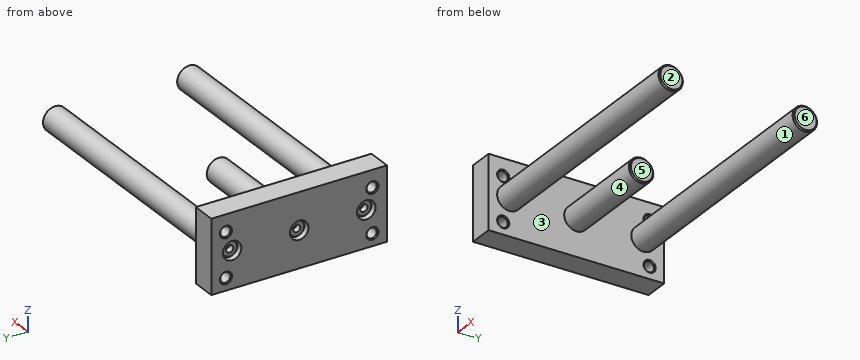
```python
from build123d import *

# Parameters (mm, degrees)
SKETCH1_W           = 30
SKETCH1_H           = 72
BOSS_EXTRUDE1_DEPTH = 10


with BuildPart() as part:
    # Sketch1 → Boss-Extrude1 (new body)
    with BuildSketch(Plane(origin=(0, 0, 0), x_dir=(0, 0, -1), z_dir=(1, 0, 0))):
        Rectangle(SKETCH1_W, SKETCH1_H)
    extrude(amount=BOSS_EXTRUDE1_DEPTH)

    # Sketch2 → Cut-Revolve1 (revolve, cut)
    with BuildSketch(Plane(origin=(0, 30, 0), x_dir=(-1, 0, 0), z_dir=(0, 1, 0)), mode=Mode.PRIVATE) as cut_revolve1_sk:
        Polygon((0, -10), (0, -12.5), (-0.433, -12.067), (-9.567, -12.067), (-10, -12.5), (-10, -10), align=None)
    revolve(cut_revolve1_sk.sketch.rotate(Axis((10, 30, -10), (-1, 0, 0)), 180), axis=Axis((10, 30, -10), (-1, 0, 0)), mode=Mode.SUBTRACT)

    # Sketch3 → Cut-Revolve2 (revolve, cut)
    with BuildSketch(Plane(origin=(0, 30, 0), x_dir=(-1, 0, 0), z_dir=(0, 1, 0)), mode=Mode.PRIVATE) as cut_revolve2_sk:
        Polygon((0, 8), (0, 5.5), (-0.433, 5.933), (-9.567, 5.933), (-10, 5.5), (-10, 8), align=None)
    revolve(cut_revolve2_sk.sketch.rotate(Axis((10, 30, 8), (-1, 0, 0)), 180), axis=Axis((10, 30, 8), (-1, 0, 0)), mode=Mode.SUBTRACT)

    # Sketch4 → Cut-Revolve3 (revolve, cut)
    with BuildSketch(Plane(origin=(0, -30, 0), x_dir=(-1, 0, 0), z_dir=(0, 1, 0)), mode=Mode.PRIVATE) as cut_revolve3_sk:
        Polygon((0, 8), (0, 5.5), (-0.433, 5.933), (-9.567, 5.933), (-10, 5.5), (-10, 8), align=None)
    revolve(cut_revolve3_sk.sketch.rotate(Axis((10, -30, 8), (-1, 0, 0)), 180), axis=Axis((10, -30, 8), (-1, 0, 0)), mode=Mode.SUBTRACT)

    # Sketch5 → Cut-Revolve4 (revolve, cut)
    with BuildSketch(Plane(origin=(0, -30, 0), x_dir=(-1, 0, 0), z_dir=(0, 1, 0)), mode=Mode.PRIVATE) as cut_revolve4_sk:
        Polygon((0, -10), (0, -12.5), (-0.433, -12.067), (-9.567, -12.067), (-10, -12.5), (-10, -10), align=None)
    revolve(cut_revolve4_sk.sketch.rotate(Axis((10, -30, -10), (-1, 0, 0)), 180), axis=Axis((10, -30, -10), (-1, 0, 0)), mode=Mode.SUBTRACT)

    # Sketch6 → Cut-Revolve5 (revolve, cut)
    with BuildSketch(Plane(origin=(0, 27.5, 0), x_dir=(-1, 0, 0), z_dir=(0, 1, 0)), mode=Mode.PRIVATE) as cut_revolve5_sk:
        Polygon((0, 0), (0, -3.8), (-5.555555556, -3.8), (-5.555555556, -3.5), (-2.055555556, -3.5), (-1.555555556, -3), (-1.555555556, -1.5), (-4.155555556, -1.5), (-5.021580959, 0), align=None)
    revolve(cut_revolve5_sk.sketch.rotate(Axis((5.021580959, 27.5, 0), (-1, 0, 0)), 180), axis=Axis((5.021580959, 27.5, 0), (-1, 0, 0)), mode=Mode.SUBTRACT)

    # Sketch7 → Cut-Revolve6 (revolve, cut)
    with BuildSketch(Plane(origin=(0, 0, 0), x_dir=(-1, 0, 0), z_dir=(0, 1, 0)), mode=Mode.PRIVATE) as cut_revolve6_sk:
        Polygon((0, 0), (0, -3.8), (-5.555555556, -3.8), (-5.555555556, -3.5), (-2.055555556, -3.5), (-1.555555556, -3), (-1.555555556, -1.5), (-4.155555556, -1.5), (-5.021580959, 0), align=None)
    revolve(cut_revolve6_sk.sketch.rotate(Axis((5.021580959, 0, 0), (-1, 0, 0)), 180), axis=Axis((5.021580959, 0, 0), (-1, 0, 0)), mode=Mode.SUBTRACT)

    # Sketch8 → Cut-Revolve7 (revolve, cut)
    with BuildSketch(Plane(origin=(0, -27.5, 0), x_dir=(-1, 0, 0), z_dir=(0, 1, 0)), mode=Mode.PRIVATE) as cut_revolve7_sk:
        Polygon((0, 0), (0, -3.8), (-5.555555556, -3.8), (-5.555555556, -3.5), (-2.055555556, -3.5), (-1.555555556, -3), (-1.555555556, -1.5), (-4.155555556, -1.5), (-5.021580959, 0), align=None)
    revolve(cut_revolve7_sk.sketch.rotate(Axis((5.021580959, -27.5, 0), (-1, 0, 0)), 180), axis=Axis((5.021580959, -27.5, 0), (-1, 0, 0)), mode=Mode.SUBTRACT)

    # Sketch9 → Revolve1 (revolve)
    with BuildSketch(Plane(origin=(0, 0, 0), x_dir=(-1, 0, 0), z_dir=(0, 1, 0)), mode=Mode.PRIVATE) as revolve1_sk:
        Polygon((-10, 0), (-10, -5), (-51.5, -5), (-52, -4.5), (-52, 0), align=None)
    revolve(revolve1_sk.sketch.rotate(Axis((52, 0, 0), (-1, 0, 0)), 180), axis=Axis((52, 0, 0), (-1, 0, 0)))

    # Sketch10 → Revolve2 (revolve)
    with BuildSketch(Plane(origin=(0, -27.5, 0), x_dir=(-1, 0, 0), z_dir=(0, 1, 0)), mode=Mode.PRIVATE) as revolve2_sk:
        Polygon((-10, 0), (-10, -5), (-113.5, -5), (-114, -4.5), (-114, 0), align=None)
    revolve(revolve2_sk.sketch.rotate(Axis((114, -27.5, 0), (-1, 0, 0)), 180), axis=Axis((114, -27.5, 0), (-1, 0, 0)))

    # Sketch11 → Revolve3 (revolve)
    with BuildSketch(Plane(origin=(0, 27.5, 0), x_dir=(-1, 0, 0), z_dir=(0, 1, 0)), mode=Mode.PRIVATE) as revolve3_sk:
        Polygon((-10, 0), (-10, -5), (-113.5, -5), (-114, -4.5), (-114, 0), align=None)
    revolve(revolve3_sk.sketch.rotate(Axis((114, 27.5, 0), (-1, 0, 0)), 180), axis=Axis((114, 27.5, 0), (-1, 0, 0)))


solid = part.part
```
Geometry: final body of the model. Coordinates: model frame, mm. Face numbers are marked on the shaded views. A direction names the side the tool comes from. Round coordinates to 2 decimals unless told otherwise and drop trailing zeros. Loops run counter-clockwise (first coordinate to the right, second up) from the corner with the lowest first, then second, coordinate; pieces in that order, holes last. Notation, with made-up numbers: (37.25, 40) -> (69.25, 40) arc R24 ccw to (69.25, 70) -> close; hole circle Ø4 at (71, 21.25). An arc over 180 degrees is marked (long way). Write each question's results on one line, items separated by ' | '.
Item 1: Cut plane C-C on x = 42. Return the cut outline in (y, z), and give its area (3 significant figures).
Answers below:
outline: circle Ø10 at (-27.5, 0); circle Ø10 at (0, 0); circle Ø10 at (27.5, 0) | area: 236 mm²
Item 2: Line query: probe 1 along Y at (x, z) = (4.25, 8); probe 2 along Z at (x, y) = (2, 27); probe 3 along Y at (x, z) = (47, 1.25). Output: solid intervals per line, ascending. Write a range as [from, to].
Answers below:
probe 1: y = [-36, -32.07], [-27.93, 27.93], [32.07, 36] | probe 2: z = [-15, -3.77], [-3.41, -1.41], [1.41, 3.41], [3.77, 15] | probe 3: y = [-32.34, -22.66], [-4.84, 4.84], [22.66, 32.34]
Item 3: Pull-direction query (Y, two-part tool) for the marked faces 1, 2 and 3; classes: pulls with the +Y half, pulls with the -Y half, needs draft (parallel to the pull), parting line crosses it, or undercut.
Answers below:
face 1: undercut | face 2: needs draft | face 3: undercut
Item 4: Set-up query: the marked faces 4, 5 and 6. Return all of +Z, -Z, +X, -X, +Y, -Y with unobstructed straight access to the full face (end or side cutting, diameter ignored); none if empty.
Answers below:
face 4: +X | face 5: +Z, -Z, +X | face 6: +Z, -Z, +X, +Y, -Y
Item 5: Cut plane A-A on z = -10. Return the cut outline in (x, y).
Answers below:
outline: (0, -36) -> (10, -36) -> (10, -32.5) -> (9.57, -32.07) -> (0.43, -32.07) -> (0, -32.5) -> close; (0, -27.5) -> (0.43, -27.93) -> (9.57, -27.93) -> (10, -27.5) -> (10, 27.5) -> (9.57, 27.93) -> (0.43, 27.93) -> (0, 27.5) -> close; (0, 32.5) -> (0.43, 32.07) -> (9.57, 32.07) -> (10, 32.5) -> (10, 36) -> (0, 36) -> close
Item 6: Cut plane B-B on x = 71. Return the cut outline in (y, z).
Answers below:
outline: circle Ø10 at (-27.5, 0); circle Ø10 at (27.5, 0)
Item 7: Cut plane D-D on y = 13.5. Return the cut outline in (x, z), and give its area (3 significant figures).
Answers below:
outline: (0, -15) -> (10, -15) -> (10, 15) -> (0, 15) -> close | area: 300 mm²
Item 8: Pin query (flat end, axial travel): pin 1 Ø1.8 at (y, z) = (-29, 0.5) entering from -X; pin 2 Ø4 at (y, z) = (0, 0) entering from +X; pin 3 Ø2.5 at (y, z) = (-30, 8) entering from +X; pin 4 Ø12 at (x, y) = (98.5, -18.5) entering from -Z. Return the tip coordinate at first contact, or that it passes through.
Answers below:
pin 1: stops at x = 1.56 | pin 2: stops at x = 52 | pin 3: passes through | pin 4: stops at z = -4
